The listing builds one solid part. Answer for the finished solid, in the listing's coordinates (mm). Round coordinates to 2 decimals unless told otherwise and drop trailing zeros. Order: outer loops, then holes, each group sorted by start corner. A loop starts at its lowest first (then second) coordinate and runs counter-clockwise, first axis right, second up. Notation, with made-up numbers: (-33, 46.5) -> (18, 46.5) arc R20 ccw to (18, 79.5) -> close; hole circle Ø2 at (8, -7). An arc over 180 degrees is marked (long way). Return JSON: item names as keys, results as strings. Group by question number.
(1) Each of these flat-tipped pins is pushed along its axis until it touches: pin 1 (2 mm diameter, centred on y = 45, z = 2.5, fed in from -X); pin 2 (1 mm diameter, centred on x = 25.5, z = 1.5, fed in from -Y); pin 3 (1.2 mm diameter, centred on x = -172, z = 1, fed in from +Y). Where does it stop, or does it pass through?
(2) The part is cut by section D-D (y = 25.5). Determine the outline of the cut face in (x, z).
(3) Consider line 1 (X direction, y = -113, z = 1.8); line 2 (X direction, y = 83, z = 1.05); line 3 (Y direction, x = -187, z = 3.4). Determine where each line is inside the solid, lowest interval first. Write a range as [from, to].
(4) The part is cut by section A-A (y = -135.5). Determine the outline of the cut face in (x, z).
(5) The part is cut by section C-C (x = -167). Determine the outline of the cut face in (y, z).
(6) The part is cut by section B-B (z = 3.05). Determine the outline of the cut face in (x, y), plus the area to 3 significant figures.
from build123d import *

# Parameters (mm, degrees)
F0_W     = 1
F0_H     = 6
F0_W_2   = 96.5
F1_DEPTH = 4


with BuildPart() as f1:
    # F0 (on Top) → F1 (new body)
    with BuildSketch(Plane.XY):
        with BuildLine():
            Line((-291.7007803917, -157.5256759562), (-55.8865144849, -157.5256759562))
            Line((-55.8865144849, -157.5256759562), (-55.8865144849, -83.4614100494))
            Line((-55.8865144849, -83.4614100494), (-55.8865144849, -77.4614100494))
            Line((-55.8865144849, -77.4614100494), (-54.8865144849, -77.4614100494))
            Line((-54.8865144849, -77.4614100494), (41.6134855151, -77.4614100494))
            Line((41.6134855151, -77.4614100494), (42.6134855151, -77.4614100494))
            Line((42.6134855151, -77.4614100494), (42.6134855151, -83.4614100494))
            Line((42.6134855151, -83.4614100494), (42.6134855151, -157.5256759562))
            Line((42.6134855151, -157.5256759562), (278.4277514219, -157.5256759562))
            Line((278.4277514219, -157.5256759562), (278.4277514219, 112.6028558574))
            Line((278.4277514219, 112.6028558574), (22.9277393461, 112.6028558574))
            ThreePointArc((22.9277393461, 112.6028558574), (6.7223803738, 98.5655061138), (1.7183407144, 77.7179538753))
            Line((1.7183407144, 77.7179538753), (1.7183407144, 17.5473609517))
            ThreePointArc((1.7183407144, 17.5473609517), (-12.6941933844, -15.5861694622), (-46.841709457, -27.3971441426))
            Line((-46.841709457, -27.3971441426), (-291.7007803917, -27.3971441426))
            Line((-291.7007803917, -27.3971441426), (-291.7007803917, -157.5256759562))
        make_face()
        with Locations((-55.3865144849, -80.4614100494)):
            Rectangle(F0_W, F0_H)
        with Locations((42.1134855151, -80.4614100494)):
            Rectangle(F0_W, F0_H)
        with Locations((-6.6365144849, -80.4614100494)):
            Rectangle(F0_W_2, F0_H)
    extrude(amount=F1_DEPTH)


solid = f1.part
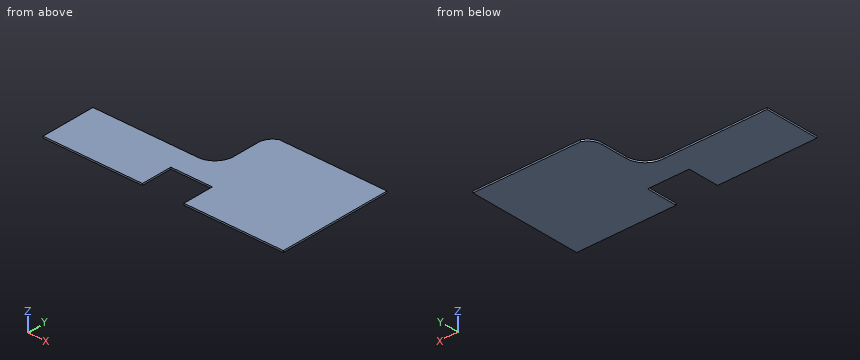
Answer below:
{
 "1": {"pin 1": "stops at x = 1.72", "pin 2": "stops at y = -83.46", "pin 3": "stops at y = -27.4"},
 "2": {"outline": "(1.72, 0) -> (278.43, 0) -> (278.43, 4) -> (1.72, 4) -> close"},
 "3": {"line 1": "x = [-291.7, -55.89], [42.61, 278.43]", "line 2": "x = [1.72, 278.43]", "line 3": "y = [-157.53, -27.4]"},
 "4": {"outline": "(-291.7, 0) -> (-55.89, 0) -> (-55.89, 4) -> (-291.7, 4) -> close; (42.61, 0) -> (278.43, 0) -> (278.43, 4) -> (42.61, 4) -> close"},
 "5": {"outline": "(-157.53, 0) -> (-27.4, 0) -> (-27.4, 4) -> (-157.53, 4) -> close"},
 "6": {"outline": "(-291.7, -157.53) -> (-55.89, -157.53) -> (-55.89, -83.46) -> (42.61, -83.46) -> (42.61, -157.53) -> (278.43, -157.53) -> (278.43, 112.6) -> (22.93, 112.6) arc R35.06 ccw to (1.72, 77.72) -> (1.72, 17.55) arc R44.94 cw to (-46.84, -27.4) -> (-291.7, -27.4) -> close", "area": "106,000 mm²"}
}
